Work out the finished part from the listing and answer in its coordinate system (mm). A direction names the side the tool comes from. Round coordinates to 2 decimals unless told otherwise and drop trailing zeros. Order: outer loops, then holes, each group sorted by start corner. A loop starts at its lowest first (then second) coordinate and runs counter-clockwise, first axis right, second up. Notation, with made-up numbers: (69.5, -31) - (107.5, -31) arc R20 ccw to (107.5, 3) - close; hole circle Ø8 at (14.25, -9.75). An arc over 180 degrees is marked (long way). Use one line per item in the form item = value. Start each with the question number.
Q1. The part is cut by section C-C on x = 24. Determine the outline of the cut face in (y, z), plus the area to 3 significant figures.
Q2. For a pull along X with two mould halves and no side action, classify faces 5 (the flat face through (-38, 64, 32.5)), 6 (the cylindrical face through (-37.4, 4.9, 40.5)), 7 (the cylindrical face through (41, 5.07, 41.07)) as +X half, -X half, draft (parallel to the pull), parting line (faces both ways), or undercut.
Q3. The part is cut by section D-D on z = -23. Determine the outline of the cut face in (x, y).
Q4. Which of the six approach directions +Z, -Z, +X, -X, +Y, -Y give full straight-line access (tool end or side, diameter ignored) to faces 1 (the flat face through (-32.5, 64, 38)), 2 (the flat face through (32.5, 64, 38)), 3 (the flat face through (37, 64, -33)), 4 (the flat face through (-38, 64, -32.5))?
Q5. Given P1, Ø5, axis at x = -39, y = 42, coming from the -Z side; P2, Ø3, axis at y = 41.5, z = 35.5, coming from the -X side; P3, Ø2, axis at x = -23.5, z = 20.5, coming from the -Y side; P4, Ø3.5, axis at x = -37.5, z = -37.5, coming from the +Y side, each flat-ended and moving along its own axis, determine where each tip first touches the part or whether it passes through.
Q6. The part is cut by section A-A on y = 46.5. Determine the outline of the cut face in (x, z).
Q7. Find the intervals of material crossed by line 1 (X direction, y = 3.75, z = -37.5); line 2 (Z direction, x = 37, y = 5); line 3 (Z direction, x = 39.5, y = 52), in increasing order. Write a range as [from, to].
Q8. The part is cut by section B-B on z = 0. Determine the outline of the cut face in (x, y), plus the area to 3 significant figures.
from build123d import *

# Parameters (mm, degrees)
CROQUIS1_W              = 85
CROQUIS1_H              = 85
SALIENTE_EXTRUIR1_DEPTH = 117
CORTAR_EXTRUIR1_START   = 10
CROQUIS2_W              = 10
CROQUIS2_H              = 10
CROQUIS2_H_2            = 9.5
CORTAR_EXTRUIR1_DEPTH   = 117
CROQUIS3_R              = 31
CORTAR_EXTRUIR2_DEPTH   = 2
CROQUIS4_R              = 8
SALIENTE_EXTRUIR2_DEPTH = 36
CROQUIS7_R              = 3
CORTAR_EXTRUIR3_DEPTH   = 10
REDONDEO7_R             = 5


with BuildPart() as part:
    # Croquis1 → Saliente-Extruir1 (new body)
    with BuildSketch(Plane(origin=(0, 0, 0), x_dir=(1, 0, 0), z_dir=(0, 1, 0))):
        Rectangle(CROQUIS1_W, CROQUIS1_H)
    extrude(amount=SALIENTE_EXTRUIR1_DEPTH)

    # Croquis2 → Cortar-Extruir1 (cut)
    with BuildSketch(Plane(origin=(0, 117, 0), x_dir=(1, 0, 0), z_dir=(0, 1, 0)).offset(CORTAR_EXTRUIR1_START)):
        with Locations((-37.5, 37.5)):
            Rectangle(CROQUIS2_W, CROQUIS2_H)
        with Locations((37.5, 37.75)):
            Rectangle(CROQUIS2_W, CROQUIS2_H_2)
        with Locations((-37.5, -37.5)):
            Rectangle(CROQUIS2_W, CROQUIS2_H)
        with Locations((37.5, -37.5)):
            Rectangle(CROQUIS2_W, CROQUIS2_H)
    extrude(amount=-CORTAR_EXTRUIR1_DEPTH, mode=Mode.SUBTRACT)

    # Croquis3 → Cortar-Extruir2 (cut)
    with BuildSketch(Plane.XZ):
        with Locations(Location((0, 0, 0), (0, 0, 270))):
            Circle(CROQUIS3_R)
    extrude(amount=-CORTAR_EXTRUIR2_DEPTH, mode=Mode.SUBTRACT)

    # Croquis4 → Saliente-Extruir2 (add)
    with BuildSketch(Plane.XZ.offset(-2)):
        with Locations(Location((0, 0, 0), (0, 0, 270))):
            Circle(CROQUIS4_R)
    extrude(amount=SALIENTE_EXTRUIR2_DEPTH)

    # Croquis7 → Cortar-Extruir3 (cut)
    with BuildSketch(Plane.XZ):
        with Locations(Location((37.5, -37.5, 0), (0, 0, 270))):
            Circle(CROQUIS7_R)
        with Locations(Location((-37.5, -37.5, 0), (0, 0, 270))):
            Circle(CROQUIS7_R)
        with Locations(Location((-37.5, 37.5, 0), (0, 0, 270))):
            Circle(CROQUIS7_R)
        with Locations(Location((37.5, 37.5, 0), (0, 0, 270))):
            Circle(CROQUIS7_R)
    extrude(amount=-CORTAR_EXTRUIR3_DEPTH, mode=Mode.SUBTRACT)

    # Redondeo7
    redondeo7_edges = [part.edges().sort_by_distance(p)[0] for p in [
        (42.5, 5, 42.5),
        (-42.5, 5, 42.5),
        (-42.5, 5, -42.5),
        (42.5, 5, -42.5),
    ]]
    fillet(redondeo7_edges, radius=REDONDEO7_R)


solid = part.part
Found:
q1.outline = (0, -42.5) - (117, -42.5) - (117, 42.5) - (0, 42.5) - (0, 19.62) - (2, 19.62) - (2, -19.62) - (0, -19.62) - close
q1.area = 9,870 mm²
q2.face_5 = draft
q2.face_6 = undercut
q2.face_7 = +X half
q3.outline = (-42.5, 0) - (-20.78, 0) - (-20.78, 2) - (20.78, 2) - (20.78, 0) - (42.5, 0) - (42.5, 117) - (-42.5, 117) - close
q4.face_1 = +Z, -X, +Y
q4.face_2 = +Z, +X, +Y
q4.face_3 = -Z, +X, +Y
q4.face_4 = -Z, -X, +Y
q5.P1 = -32.5
q5.P2 = -32.5
q5.P3 = 0
q5.P4 = through
q6.outline = (-42.5, -32.5) - (-32.5, -32.5) - (-32.5, -42.5) - (32.5, -42.5) - (32.5, -33) - (42.5, -33) - (42.5, 32.5) - (32.5, 32.5) - (32.5, 42.5) - (-32.5, 42.5) - (-32.5, 32.5) - (-42.5, 32.5) - close
q7.line_1 = [-42.5, -40.5], [-34.5, 34.5], [40.5, 42.5]
q7.line_2 = [-42.5, -40.46], [-34.54, 34.54], [40.46, 42.5]
q7.line_3 = [-33, 32.5]
q8.outline = (-42.5, 0) - (-31, 0) - (-31, 2) - (-8, 2) - (-8, -34) - (8, -34) - (8, 2) - (31, 2) - (31, 0) - (42.5, 0) - (42.5, 117) - (-42.5, 117) - close
q8.area = 10,400 mm²
